Design review of the part built by this model. Coordinates are the model's own, in mm. A direction names the side the tool comes from. Round coordinates to 2 decimals unless told otherwise and drop trailing zeros. Loops run counter-clockwise (first coordinate to the right, second up) from the corner with the lowest first, then second, coordinate; pieces in that order, holes last. Notation, with made-up numbers: (87.5, 23) -> (94.5, 23) arc R11 ccw to (94.5, 39) -> close; hole circle Ø4 at (-17, 23). An arc over 180 degrees is marked (long way). Write each question's results on one line, items separated by ' | '. Start each with the question number.
from build123d import *

# Parameters (mm, degrees)
SKETCH3_W           = 1.5
SKETCH3_H           = 2.5
BOSS_EXTRUDE1_DEPTH = 4
SKETCH4_R           = 6
BOSS_EXTRUDE2_DEPTH = 4.5
BOSS_EXTRUDE3_DEPTH = 14


with BuildPart() as part:
    # Sketch2 → Revolve1 (revolve)
    with BuildSketch(Plane(origin=(0, 0, 0), x_dir=(1, 0, 0), z_dir=(0, 1, 0))):
        Polygon((0, -54), (0, 0), (17.75, 0), (17.75, -31), (18.5, -31), (18.5, -54), align=None)
    revolve(axis=Axis((0, 0, 54), (0, 0, -1)))

    # Sketch3 → Boss-Extrude1 (add)
    with BuildSketch(Plane(origin=(0, 0, 0), x_dir=(-1, 0, 0), z_dir=(0, 0, -1))):
        with Locations((-12.5, 0)):
            Rectangle(SKETCH3_W, SKETCH3_H)
        with Locations((12.5, 0)):
            Rectangle(SKETCH3_W, SKETCH3_H)
    extrude(amount=BOSS_EXTRUDE1_DEPTH)

    # Sketch4 → Boss-Extrude2 (add)
    with BuildSketch(Plane.XY.offset(54)):
        with Locations((0, -7)):
            Circle(SKETCH4_R)
        with BuildLine():
            Line((-1.658312395, -9.5), (1.658312395, -9.5))
            ThreePointArc((1.658312395, -9.5), (0, -4), (-1.658312395, -9.5))
        make_face(mode=Mode.SUBTRACT)
    extrude(amount=BOSS_EXTRUDE2_DEPTH)

    # Sketch4<2> → Boss-Extrude3 (add)
    with BuildSketch(Plane.XY.offset(54)):
        with BuildLine():
            Line((-1.658312395, -9.5), (1.658312395, -9.5))
            ThreePointArc((1.658312395, -9.5), (0, -4), (-1.658312395, -9.5))
        make_face()
    extrude(amount=BOSS_EXTRUDE3_DEPTH)


solid = part.part
1) The part is to be moulded in two halves that separate along X. For faces 5 (the face through (-13.25, 0, -2)), 6 (the face through (-12, -1.25, -2)), 7 (the face through (11.75, 0, -2)), 8 (the face through (-4.01, 18.06, 42.66)), say which applies: +X half, -X half, draft (parallel to the pull), parting line (faces both ways), or undercut.
2) To check wall thickness, follow line 1 (Z direction, x = -6.5, y = -14); line 2 (Y direction, x = 0.5, z = 46); line 3 (Z direction, x = -12, y = 0). State the ranges of each line that lie inside material, in increasing order. Write a range as from..to.
3) Insertion check: pin 1 (1.2 mm diameter, centred on y = 0, z = -2.5, fed in from -X); pin 2 (6 mm diameter, centred on x = -4, y = 1.5, fed in from +Z); pin 3 (4 mm diameter, centred on y = 12.5, z = 27.5, fed in from +X); pin 4 (12 mm diameter, centred on x = 3.5, y = -1.5, fed in from +Z). Each pin has a flat end and moves straight along its axis. Give the tip position at first contact, or say it passes through.
4) Take a section at B-B (x = 0). Write out the cut boundary in (y, z).
5) For faces 1 (the face through (-6, -7, 56)), 2 (the face through (-11.75, 0, -2)), 3 (the face through (-3.848, 17.328, 15.717)), 4 (the face through (13, 1.25, -2)), list the 3-axis set-ups (+Z, -Z, +X, -X, +Y, -Y) from which the entire face can be reached by the end or side of a thin tool; tool diameter is ignored.
6) Take a section at D-D (y = 8.5). Write out the cut boundary in (x, z).
7) Take a section at C-C (z = 50). Write out the cut boundary in (x, y).
8) Take a section at A-A (y = 0). Write out the cut boundary in (x, z).
Geometry check:
1) face 5: -X half | face 6: draft | face 7: undercut | face 8: parting line
2) line 1: z = 0..54 | line 2: y = -18.49..18.49 | line 3: z = -4..54
3) pin 1: stops at x = -13.25 | pin 2: stops at z = 54 | pin 3: stops at x = 14.31 | pin 4: stops at z = 68
4) outline: (-18.5, 31) -> (-17.75, 31) -> (-17.75, 0) -> (17.75, 0) -> (17.75, 31) -> (18.5, 31) -> (18.5, 54) -> (-1, 54) -> (-1, 58.5) -> (-4, 58.5) -> (-4, 68) -> (-9.5, 68) -> (-9.5, 58.5) -> (-13, 58.5) -> (-13, 54) -> (-18.5, 54) -> close
5) face 1: +Z | face 2: -Z, +Y, -Y | face 3: -Z | face 4: -Z, +X, -X, +Y
6) outline: (-16.43, 31) -> (-15.58, 31) -> (-15.58, 0) -> (15.58, 0) -> (15.58, 31) -> (16.43, 31) -> (16.43, 54) -> (-16.43, 54) -> close
7) outline: circle Ø37 at (0, 0)
8) outline: (-18.5, 31) -> (-17.75, 31) -> (-17.75, 0) -> (-13.25, 0) -> (-13.25, -4) -> (-11.75, -4) -> (-11.75, 0) -> (11.75, 0) -> (11.75, -4) -> (13.25, -4) -> (13.25, 0) -> (17.75, 0) -> (17.75, 31) -> (18.5, 31) -> (18.5, 54) -> (-18.5, 54) -> close
